For this review, take the finished solid that the model builds, in its own axes (mm). A direction names the side the tool comes from. Round coordinates to 2 decimals unless told otherwise and drop trailing zeros. Loops run counter-clockwise (first coordinate to the right, second up) from the corner with the lowest first, then second, coordinate; pieces in that order, holes last. Notation, with made-up numbers: (35.25, 81.5) -> (50.25, 81.5) arc R26 ccw to (50.25, 113.5) -> close; hole circle Ø6 at (-3.5, 78.5). An arc over 180 degrees is marked (long way). Write each question's results on one line, items separated by ' | '.
```python
from build123d import *

# Parameters (mm, degrees)
SKETCH1_R                     = 38
SKETCH1_R_2                   = 33
BOSS_EXTRUDE1_DEPTH           = 20
BOSS_EXTRUDE2_START           = 20
SKETCH4_R                     = 38
SKETCH4_R_2                   = 6
BOSS_EXTRUDE2_DEPTH           = 20
CHAMFER1_SIZE                 = 10
CHAMFER1_SIZE_2               = 27.474774195
SKETCH5_R                     = 38
SKETCH5_R_2                   = 29
CUT_EXTRUDE1_DEPTH            = 3
LPATTERN1_COUNT               = 4
LPATTERN1_PITCH               = 5
HOLE_FOR_4_300_SC_NUTS_SP_1_D = 4.2164
CIRPATTERN1_COUNT             = 3


with BuildPart() as part:
    # Sketch1 → Boss-Extrude1 (new body)
    with BuildSketch(Plane.XY):
        Circle(SKETCH1_R)
        Circle(SKETCH1_R_2, mode=Mode.SUBTRACT)
    extrude(amount=BOSS_EXTRUDE1_DEPTH)

    # Sketch4 → Boss-Extrude2 (add)
    with BuildSketch(Plane(origin=(0, 0, 0), x_dir=(-1, 0, 0), z_dir=(0, 0, -1)).offset(BOSS_EXTRUDE2_START)):
        Circle(SKETCH4_R)
        Circle(SKETCH4_R_2, mode=Mode.SUBTRACT)
    extrude(amount=-BOSS_EXTRUDE2_DEPTH)

    # Chamfer1
    # the kernel refuses this chamfer: 27.474774195, 10 mm, written as the material it takes off along each edge
    with BuildSketch(Plane(origin=(0, 0, 0), x_dir=(-1, 0, 0), z_dir=(0, -1, 0))) as chamfer1_piece_1_section:
        Polygon((6, CHAMFER1_SIZE), (6 + CHAMFER1_SIZE_2, 0), (6, 0), align=None)
    chamfer1_piece_1 = revolve(axis=Axis((0, 0, 0), (0, 0, -1)), mode=Mode.PRIVATE)
    chamfer1_piece_1 = chamfer1_piece_1 & Plane(origin=(0, 0, -5.040402046), x_dir=(1, 0, 0), z_dir=(0, 0, -1)) * Cylinder(33, 134, mode=Mode.PRIVATE)
    add(chamfer1_piece_1, mode=Mode.SUBTRACT)

    # Sketch5 → Cut-Extrude1 (cut)
    with BuildSketch(Plane(origin=(0, 0, -20), x_dir=(-1, 0, 0), z_dir=(0, 0, -1))):
        Circle(SKETCH5_R)
        Circle(SKETCH5_R_2, mode=Mode.SUBTRACT)
    cut_extrude1 = extrude(amount=-CUT_EXTRUDE1_DEPTH, mode=Mode.SUBTRACT)

    # LPattern1: Cut-Extrude1 ×4
    with Locations(*[(0, 0, i * LPATTERN1_PITCH) for i in range(1, LPATTERN1_COUNT)]):
        add(cut_extrude1, mode=Mode.SUBTRACT)

    # Hole for #4 300® SC Nuts (SP)1 (through all)
    with Locations(Plane.XY.offset(20)):
        with Locations((0, 35.5)):
            hole_for_4_300_sc_nuts_sp_1 = Hole(HOLE_FOR_4_300_SC_NUTS_SP_1_D / 2)

    # CirPattern1: Hole for #4 300® SC Nuts (SP)1 ×3 about axis
    cirpattern1_axis = Axis((0, 0, 0), (0, 0, 1))
    for i in range(1, CIRPATTERN1_COUNT):
        add(hole_for_4_300_sc_nuts_sp_1.rotate(cirpattern1_axis, i * 360 / CIRPATTERN1_COUNT), mode=Mode.SUBTRACT)


solid = part.part
```
1. Tool access review of faces 1 (the face through (-8.3, -28, -17)), 2 (the face through (-8.3, -28, -7)), 3 (the face through (28.73, -17.12, -6.01)): name each direction out of +Z, -Z, +X, -X, +Y, -Y from which nothing blocks a thin tool from reaching the whole face with its end or side.
Values found:
face 1: -Z | face 2: none | face 3: +Z, -Z
2. Consider section D-D (z = -8.5). State the section outline as (x, y) points.
Values found:
outline: circle Ø58 at (0, 0); hole circle Ø20.24 at (0, 0)
3. Draft analysis for pull direction Y (two halves, no side actions). For faces 4 (the face through (0.27, 37.59, -16.01)), 5 (the face through (-13.38, -25.73, -8.52)), 6 (the face through (0, 7, -20)), state which applies: released by +Y, released by -Y, zero draft, split by the parting line, or undercut.
Values found:
face 4: undercut | face 5: split by the parting line | face 6: zero draft
4. Consider section A-A (y = 35.5). Give the number of separate pieces and of enclosed holes in the cut face, plus the area to 3 significant figures.
Values found:
separate pieces: 8 | enclosed holes: 0 | area: 641 mm2
5. For pin 1 (8 mm diameter, centred on y = 24, z = -4.5, fed in from +X); pin 2 (2.5 mm diameter, centred on x = 30.74, y = -17.75, fed in from +Z); pin 3 (5 mm diameter, centred on x = 15.5, z = -15, fed in from -Y); pin 4 (6.5 mm diameter, centred on x = 0, y = 35.5, fed in from -Z), all flat-tipped, find the tip position at first contact; note any pin that passes through.
Values found:
pin 1: stops at x = 32.29 | pin 2: passes through | pin 3: stops at y = -35.71 | pin 4: stops at z = -17
6. To check wall thickness, follow probe 1 along Z at (x, y) = (10.5, 33); probe 2 along X at (y, z) = (-17, -11); probe 3 along Z at (x, y) = (-31.5, 9). State the ranges of each line that lie inside material, in increasing order.
Values found:
probe 1: z = -17 to -15, -12 to -10, -7 to -5, -2 to 20 | probe 2: x = -33.99 to -32.71, -28.77 to 28.77, 32.71 to 33.99 | probe 3: z = -17 to -15, -12 to -10, -7 to -5, -2 to -0.26
